Check sheet for the modelled part. Datum: model origin and axes. Units: mm. A direction names the side the tool comes from. Give positions to 0.01 mm unless a question says otherwise; leave off trailing zeros. Order: outer loops, then holes, each group sorted by start corner. A loop starts at its lowest first (then second) coordinate and runs counter-clockwise, first axis right, second up.
Autodesk Inventor part; units mm, degrees
ref_plane "YZ Plane" through (0, 0, 0) normal (1, 0, 0) x (0, 1, 0)
ref_plane "XZ Plane" through (0, 0, 0) normal (0, 1, 0) x (-1, 0, 0)
ref_plane "XY Plane" through (0, 0, 0) normal (0, 0, 1) x (1, 0, 0)
sketch "Sketch1" plane through (0, 0, 0) normal (0, 1, 0) x (-1, 0, 0)
  line L0 (9.98, 16.98) -> (-9.98, 16.98)
  line L1 (-9.98, 16.98) -> (-9.98, -16.98)
  line L2 (-9.98, -16.98) -> (9.98, -16.98)
  line L3 (9.98, -16.98) -> (9.98, 16.98)
  line L4 (9.98, 16.98) -> (-9.98, -16.98) construction
  line L5 (-9.98, 16.98) -> (9.98, -16.98) construction
  point P0 (0, 0)
  dimension "d0" = 33.96
  dimension "d1" = 19.96
extrude "arm-wall" add sketch "Sketch1" along normal blind 3
sketch "Sketch2" plane through (0, 3, 0) normal (0, 1, 0) x (1, 0, 0)
  line L0 (-8, -16.98) -> (8, -16.98)
  line L1 (8, -16.98) -> (8, 15.98)
  line L2 (8, 15.98) -> (-8, 15.98)
  line L3 (-8, 15.98) -> (-8, -16.98)
  line L4 (-8, -16.98) -> (8, 15.98) construction
  line L5 (8, -16.98) -> (-8, 15.98) construction
  line L6 (0, 23.772) -> (0, -23.772)
  line L7 (9.98, 16.98) -> (-9.98, 16.98)
  line L8 (-9.98, -16.98) -> (9.98, -16.98)
  point P0 (0, 0)
  point P1 (0, -0.5)
  point P2 (0, -0.5)
  dimension "d4" = 16
  dimension "d5" = 1
extrude "slot" cut sketch "Sketch2" against normal blind 2
sketch "Sketch3" plane through (0, 0, 0) normal (0, -1, 0) x (1, 0, 0)
  circle A0 centre (0, 0) radius 2.5
  dimension "d12" = 5
extrude "Extrusion3" cut sketch "Sketch3" against normal blind 2
sketch "Sketch4" plane through (-9.98, 0, 16.98) normal (0, 0, 1) x (1, 0, 0)
  line L0 (1.98, 1) -> (0.88, 1)
  line L1 (0.88, 1) -> (0.88, 2.1)
  line L2 (0.88, 2.1) -> (1.98, 2.1)
  line L3 (1.98, 2.1) -> (1.98, 1)
  line L4 (17.98, 1) -> (19.08, 1)
  line L5 (19.08, 1) -> (19.08, 2.1)
  line L6 (19.08, 2.1) -> (17.98, 2.1)
  line L7 (17.98, 2.1) -> (17.98, 1)
  point P0 (9.98, 0)
  dimension "d15" = 1.1
  dimension "d16" = 1.1
  dimension "d17" = 1.1
  dimension "d18" = 1.1
extrude "Extrusion4" cut sketch "Sketch4" against normal up to surface (32.96 mm away)
sketch "Sketch5" plane through (9.98, 0, -16.98) normal (0, 0, -1) x (-1, 0, 0)
  line L0 (9.98, 5.9286) -> (9.98, -4.0714)
  line L1 (0, 0) -> (19.96, 0)
  line L2 (3.48, 3) -> (16.48, 3)
  line L3 (16.48, 3) -> (16.48, 1)
  line L4 (16.48, 1) -> (3.48, 1)
  line L5 (3.48, 1) -> (3.48, 3)
  line L6 (0, 3) -> (19.96, 3)
  point P0 (9.98, 0)
  point P1 (9.98, 0)
  dimension "d21" = 10
  dimension "d22" = 1
  dimension "d23" = 13
extrude "Extrusion5" cut sketch "Sketch5" against normal up to next
equation "\"d2\" = armthick"
equation "\"d4\" = adapterh"
equation "\"d5\" = -0.5 * adapterw + 0.5 * armw"
equation "\"d6\" = armslotd"
equation "\"d15\" = d16"
equation "\"d17\" = d15"
equation "\"d18\" = d16"
equation "\"printer3dtolerance\" = 0.1"
equation "\"wallw\" = 42"
equation "\"wallh\" = 44"
equation "\"cornerrad\" = 2"
equation "\"baseextra\" = 2"
equation "\"wall1_thick\" = 8"
equation "\"wall2_thick\" = 6.4"
equation "\"wall3_thick\" = 4"
equation "\"wall1slot\" = 8.1"
equation "\"wall2slot\" = 6.5"
equation "\"wall3slot\" = 4.1"
equation "\"gap2\" = 28"
equation "\"baseh\" = 79"
equation "\"basew\" = 44"
equation "\"base_thick\" = 6"
equation "\"base_slots_depth\" = 4"
equation "\"servobigcircledia\" = 11.6"
equation "\"servosmallcircledia\" = 5.9"
equation "\"servo9gw\" = 22.8"
equation "\"servomounth\" = 4"
equation "\"servomountsquare\" = 4"
equation "\"servopolygonr\" = 6.1"
equation "\"servopolygonl\" = 5.9"
equation "\"distancefrombottom\" = 34"
equation "\"distancefromleft\" = 22"
equation "\"wall3slotd\" = 2"
equation "\"wall3slotw\" = 36"
equation "\"adapterh\" = 16"
equation "\"adapterw\" = 32"
equation "\"armw\" = 34"
equation "\"armslotd\" = 2"
equation "\"armthick\" = 3"
equation "\"fanhb\" = 11"
equation "\"fanhs\" = 9.6"
equation "\"adapterwallslotd\" = 2"
equation "\"adapterwallthick\" = 6"
equation "\"armhornthick\" = 3"
equation "\"hornscrewholed\" = 2"
equation "\"hornscrewheadd\" = 3"
equation "\"hornthick\" = 1.5"
properties part number "arm-slot"
(1) Thickness scan on L1, parallel to X at y = 2.4, z = -14.5; L2, parallel to Z at x = 0, y = 0.85; L3, parallel to Y at x = -8.5, z = -10.5. Record the ranges inside material, lowest first.
(2) Sectioned sample at B-B (x = 0). Enter the section's corners in (y, z), plus the area to 3 significant figures.
(3) Tool access check on faces 1 (the face through (-6.5, 2, -16.5)), 2 (the face through (8, 2.6, 0.7)), 3 (the face through (9.98, 1, 0)), 4 (the face through (-8.6, 2.1, 0.7)). Record the directions out of +Z, -Z, +X, -X, +Y, -Y that give a thin tool (end or side, any length) a straight path to the whole face; none if there is none.
(4) Sectioned sample at D-D (z = 6). Enter the section's corners in (x, y), plus the area to 3 significant figures.
(5) Go/stop test with flat-tipped pins: P1, Ø1.2, axis at x = 8.5, z = -6.5, coming from the -Y side; P2, Ø8, axis at x = 0, z = 0, coming from the +Y side. Record where each tip stops, or that it passes through.
(6) Release check for a two-part mould opening along X. For faces 5 (the face through (-9.98, 1, 0)), 6 (the face through (-0.1, 0.8, 16.98)), 7 (the face through (0, 1, -4)), 8 (the face through (8.6, 2.1, 0.7)) record: released by +X, released by -X, zero draft, split by the parting line, or undercut.
(7) Sectioned sample at A-A (y = 1.5). Enter the section's corners in (x, z).
(8) Sectioned sample at C-C (z = 0). Enter the section's corners in (x, y).
Values follow:
1. L1: x = -9.98 to -8, 8 to 9.98
1. L2: z = -16.98 to -2.5, 2.5 to 16.98
1. L3: y = 0 to 1, 2.1 to 3
2. outline: (0, -16.98) - (1, -16.98) - (1, -2.5) - (0, -2.5) - close; (0, 2.5) - (1, 2.5) - (1, 16.98) - (0, 16.98) - close
2. area: 29.0 mm2
3. face 1: +Z, -Z, +Y
3. face 2: +Z, +Y
3. face 3: +Z, -Z, +X, +Y, -Y
3. face 4: +Z
4. outline: (-9.98, 0) - (9.98, 0) - (9.98, 3) - (8, 3) - (8, 2.1) - (9.1, 2.1) - (9.1, 1) - (-9.1, 1) - (-9.1, 2.1) - (-8, 2.1) - (-8, 3) - (-9.98, 3) - close
4. area: 25.5 mm2
5. P1: stops at y = 0
5. P2: stops at y = 1
6. face 5: released by -X
6. face 6: zero draft
6. face 7: undercut
6. face 8: undercut
7. outline: (-9.98, -16.98) - (-6.5, -16.98) - (-6.5, -15.98) - (-9.1, -15.98) - (-9.1, 16.98) - (-9.98, 16.98) - close; (6.5, -16.98) - (9.98, -16.98) - (9.98, 16.98) - (9.1, 16.98) - (9.1, -15.98) - (6.5, -15.98) - close
8. outline: (-9.98, 0) - (-2.5, 0) - (-2.5, 1) - (-9.1, 1) - (-9.1, 2.1) - (-8, 2.1) - (-8, 3) - (-9.98, 3) - close; (2.5, 0) - (9.98, 0) - (9.98, 3) - (8, 3) - (8, 2.1) - (9.1, 2.1) - (9.1, 1) - (2.5, 1) - close
